from build123d import *

# Parameters (mm, degrees)
F0_W     = 844.55
F0_H     = 158.75
F1_DEPTH = 19.05
F3_R     = 9.525
F4_DEPTH = 101.6
F5_R     = 9.52499
F7_R     = 9.525
F8_DEPTH = 101.6
F9_R     = 9.52499
F10_R    = 9.52499


# Not quite as in the source:
# - a fillet or chamfer is up to 0.001 mm smaller than in the source, because OpenCascade refuses the exact size


with BuildPart() as f1:
    # F0 (on Right) → F1 (new body)
    with BuildSketch(Plane.YZ):
        Rectangle(F0_W, F0_H)
    extrude(amount=F1_DEPTH)

    # F3 (on offset) → F4 (cut)
    with BuildSketch(Plane.XZ.offset(339.725)):
        with Locations((0, 79.375)):
            Circle(F3_R)
    extrude(amount=-F4_DEPTH, mode=Mode.SUBTRACT)

    # F5 (radius 9.525 in the source; OpenCascade refuses exactly that, so slightly less here)
    f5_edges = [f1.edges().sort_by_distance(p)[0] for p in [
        (6.735192, -339.725, 72.639808),
        (6.735192, -238.125, 72.639808),
    ]]
    fillet(f5_edges, radius=F5_R)

    # F7 (on offset) → F8 (cut)
    with BuildSketch(Plane(origin=(0, 327.025, 0), x_dir=(-1, 0, 0), z_dir=(0, 1, 0))):
        with Locations((0, 79.375)):
            Circle(F7_R)
    extrude(amount=-F8_DEPTH, mode=Mode.SUBTRACT)

    # F9 (radius 9.525 in the source; OpenCascade refuses exactly that, so slightly less here)
    f9_edges = [f1.edges().sort_by_distance(p)[0] for p in [
        (6.735192, 225.425, 72.639808),
        (6.735192, 327.025, 72.639808),
    ]]
    fillet(f9_edges, radius=F9_R)

    # F10 (radius 9.525 in the source; OpenCascade refuses exactly that, so slightly less here)
    f10_edges = [f1.edges().sort_by_distance(p)[0] for p in [
        (19.05, -422.275, 0),
        (19.05, 0, 79.375),
        (19.05, 422.275, 0),
        (19.05, 0, -79.375),
    ]]
    fillet(f10_edges, radius=F10_R)


solid = f1.part
For this review, take the finished solid that the model builds, in its own axes (mm). Coordinates: 2 decimals unless noted, no trailing zeros. Order: outer loops, then holes, each group sorted by start corner. A loop starts at its lowest first (then second) coordinate and runs counter-clockwise, first axis right, second up. Notation, with made-up numbers: (51, -39.75) -> (65, -39.75) arc R24 ccw to (65, -11.75) -> close; hole circle Ø1 at (62, 13). An arc over 180 degrees is marked (long way). Return JSON: item names as keys, results as strings.
1. For line 1 (Y direction, x = 11, z = 64.5); line 2 (Z direction, x = 1.25, y = -308.5) (3 decimals); line 3 (Z direction, x = 11.25, y = 193), list the stretches that pass through material, from the lowest coordinate up. Write a range as from..to.
Answer block:
{"line 1": "-422.16..422.16", "line 2": "-79.375..69.932", "line 3": "-79.22..79.22"}
2. We need section B-B on x = 14. Write out the cut boundary in (y, z), and give its area (3 significant figures).
Answer block:
{"outline": "(-421.16, -78.26) -> (421.16, -78.26) -> (421.16, 78.26) -> (-421.16, 78.26) -> close", "area": "132,000 mm²"}
3. For pin 1 Ø1 at (x, z) = (14.5, -3.5) entering from -Y; pin 2 Ø1 at (x, y) = (13, -317) entering from -Z; pin 3 Ø8 at (x, y) = (15.5, 125.5) entering from +Z, all flat-tipped, find the tip position at first contact; note any pin that passes through.
Answer block:
{"pin 1": "y = -421.16", "pin 2": "z = -78.9", "pin 3": "z = 79.17"}
